Build history of the part. All positions in model axes, mm. A direction names the side the tool comes from. Give positions to 0.01 mm unless a question says otherwise; leave off trailing zeros. Write each loop counter-clockwise with the first axis right and the second up, starting at its lowest first coordinate (ties: lowest second). Pieces come first, ordered by that corner, then holes. Notation, with made-up numbers: (20, 11) -> (57, 11) arc R22 ccw to (57, 29) -> close; hole circle Ø11 at (35.25, 75.5). An arc over 180 degrees is marked (long way). Put each result on its own line as item: value.
from build123d import *

# Parameters (mm, degrees)
F0_R     = 1
F0_R_2   = 7.5
F1_DEPTH = 6


with BuildPart() as f1:
    # F0 (on Top) → F1 (new body)
    with BuildSketch(Plane.XY):
        Polygon((-10, 36.175396), (-16, 36.175396), (-16, 19.625396), (-21.45, 14.175396), (-21.45, -11.824604), (21.45, -11.824604), (21.45, 14.175396), (16, 19.625396), (16, 36.175396), (10, 36.175396), (10, 26.175396), (-10, 26.175396), align=None)
        with Locations((-13.526969, 7.675396)):
            Circle(F0_R, mode=Mode.SUBTRACT)
        with Locations((0, 1.175396)):
            Circle(F0_R_2, mode=Mode.SUBTRACT)
        with Locations((13.526969, 7.675396)):
            Circle(F0_R, mode=Mode.SUBTRACT)
        with Locations((-13.526969, 15.675396)):
            Circle(F0_R, mode=Mode.SUBTRACT)
        with Locations((-13.163304, 23.675396)):
            Circle(F0_R, mode=Mode.SUBTRACT)
        with Locations((-12.886655, 31.675396)):
            Circle(F0_R, mode=Mode.SUBTRACT)
        with Locations((13.526969, 15.675396)):
            Circle(F0_R, mode=Mode.SUBTRACT)
        with Locations((13.163304, 23.675396)):
            Circle(F0_R, mode=Mode.SUBTRACT)
        with Locations((12.886655, 31.675396)):
            Circle(F0_R, mode=Mode.SUBTRACT)
    extrude(amount=F1_DEPTH)


solid = f1.part
1) Pull direction X, two halves, no side cores. Call faces 1 (the flat face through (-13, 36.175, 3)), 2 (the cylindrical face through (13.033, 24.667, 2.958)), 3 (the flat face through (-21.45, 1, 3)): released by +X, released by -X, zero draft, split by the parting line, or undercut.
Filled sheet:
face 1: zero draft
face 2: undercut
face 3: released by -X
2) Slice it at B-B (x = 0). Write the cut outline in (y, z), plus the area to 3 significant figures.
Filled sheet:
outline: (-11.82, 0) -> (-6.32, 0) -> (-6.32, 6) -> (-11.82, 6) -> close; (8.68, 0) -> (26.18, 0) -> (26.18, 6) -> (8.68, 6) -> close
area: 138 mm2
3) Wall check: L1, parallel to X at y = 29.5, z = 4.05; L2, parallel to X at y = 7.5, z = 5.05; L3, parallel to X at y = 0, z = 4.3. Give the ranges that are in metal, low to high.
Filled sheet:
L1: -16 to -10, 10 to 16
L2: -21.45 to -14.51, -12.54 to -4.03, 4.03 to 12.54, 14.51 to 21.45
L3: -21.45 to -7.41, 7.41 to 21.45
4) Tool access for faces 4 (the flat face through (-16, 28, 3)), 5 (the flat face through (10, 31, 3)), 6 (the cylindrical face through (14.45, 7.29, 2.96)), 7 (the flat face through (16, 28, 3)): list every direction of +Z, -Z, +X, -X, +Y, -Y with a clear straight run to the whole face (end or side of a thin tool).
Filled sheet:
face 4: +Z, -Z, -X, +Y
face 5: +Z, -Z, +Y
face 6: +Z, -Z
face 7: +Z, -Z, +X, +Y
5) Slice it at A-A (y = 27). Write the cut outline in (x, z), plus the area to 3 significant figures.
Filled sheet:
outline: (-16, 0) -> (-10, 0) -> (-10, 6) -> (-16, 6) -> close; (10, 0) -> (16, 0) -> (16, 6) -> (10, 6) -> close
area: 72.0 mm2
6) Slice it at C-C (z = 0.6). Give the number of separate pieces and of enclosed holes in the cut face, plus the area to 3 significant figures.
Filled sheet:
separate pieces: 1
enclosed holes: 9
area: 1,450 mm2
7) Slice it at D-D (y = 21). Write the cut outline in (x, z).
Filled sheet:
outline: (-16, 0) -> (16, 0) -> (16, 6) -> (-16, 6) -> close
